```python
from build123d import *

# Parameters (mm, degrees)
SKETCH4_R           = 1.911425658
BOSS_EXTRUDE1_DEPTH = 5.6


with BuildPart() as part:
    # Sketch4 → Boss-Extrude1 (new body)
    with BuildSketch(Plane(origin=(0, 0, 0), x_dir=(1, 0, 0), z_dir=(0, 1, 0))):
        with BuildLine():
            Line((-4, -3.25), (-8.327817762, -2.730391092))
            ThreePointArc((-8.327817762, -2.730391092), (-10.75, 0), (-8.327817762, 2.730391092))
            Line((-8.327817762, 2.730391092), (-4, 3.25))
            Line((-4, 3.25), (4, 3.25))
            Line((4, 3.25), (8.327817762, 2.730391092))
            ThreePointArc((8.327817762, 2.730391092), (10.75, 0), (8.327817762, -2.730391092))
            Line((8.327817762, -2.730391092), (4, -3.25))
            Line((4, -3.25), (-4, -3.25))
        make_face()
        Circle(SKETCH4_R, mode=Mode.SUBTRACT)
    extrude(amount=BOSS_EXTRUDE1_DEPTH)


solid = part.part
```
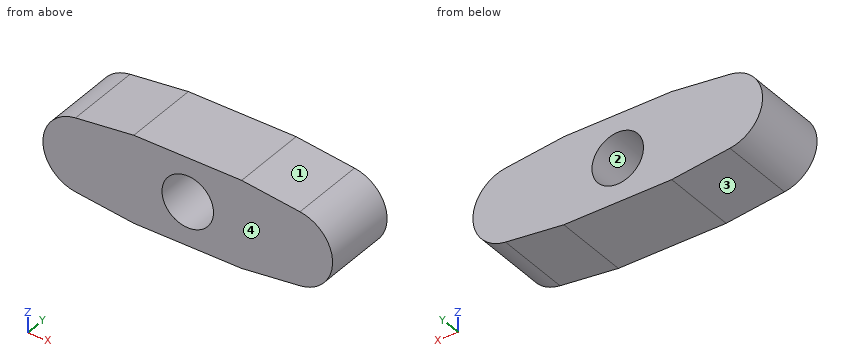
Model file for the job. Use its own axes, mm. Face numbers are marked on the shaded views. Give positions to 0.01 mm unless a question says otherwise; leave off trailing zeros. Loops run counter-clockwise (first coordinate to the right, second up) from the corner with the lowest first, then second, coordinate; pieces in that order, holes last. Notation, with made-up numbers: (32, -0.75) - (86, -0.75) arc R8 cw to (86, 7.25) - close; hole circle Ø4 at (20, -34). An arc over 180 degrees is marked (long way). One line per item, written item: value. Start each with the question number.
1. Probe L1, parallel to Z at x = 0, y = 4.1; L2, parallel to X at y = 1.65, z = 0; L3, parallel to X at y = 3.35, z = -1.25. List the from-to ranges inside material, lowest first. Write a range as from..to.
2. Slice it at A-A (x = 0). List the corners of the cut face in (y, z), plus the area to 3 significant figures.
3. Slice it at C-C (y = 0.6). List the corners of the cut face in (x, z), plus the area to 3 significant figures.
4. Pin check, flat tip, straight feed: pin 1 (2 mm diameter, centred on y = 3, z = 2, fed in from +X). Stop position of the tip, or through.
5. Pull direction X, two halves, no side cores. Call the marked faces 1, 2, 3 and 4: pulls with the +X half, pulls with the -X half, needs draft (parallel to the pull), parting line crosses it, or undercut.
6. Slice it at B-B (z = 0). List the corners of the cut face in (x, y), plus the area to 3 significant figures.
7. Slice it at D-D (z = 2.5). List the corners of the cut face in (x, y).
Solution:
1. L1: z = -3.25..-1.91, 1.91..3.25
1. L2: x = -10.75..-1.91, 1.91..10.75
1. L3: x = -10.45..-1.45, 1.45..10.45
2. outline: (0, -3.25) - (5.6, -3.25) - (5.6, -1.91) - (0, -1.91) - close; (0, 1.91) - (5.6, 1.91) - (5.6, 3.25) - (0, 3.25) - close
2. area: 15.0 mm^2
3. outline: (-8.33, -2.73) - (-4, -3.25) - (4, -3.25) - (8.33, -2.73) arc R2.75 ccw to (8.33, 2.73) - (4, 3.25) - (-4, 3.25) - (-8.33, 2.73) arc R2.75 ccw to start; hole circle Ø3.82 at (0, 0)
3. area: 112 mm^2
4. pin 1: stops at x = 10.56
5. face 1: pulls with the +X half
5. face 2: undercut
5. face 3: pulls with the -X half
5. face 4: needs draft
6. outline: (-10.75, 0) - (-1.91, 0) - (-1.91, 5.6) - (-10.75, 5.6) - close; (1.91, 0) - (10.75, 0) - (10.75, 5.6) - (1.91, 5.6) - close
6. area: 99.0 mm^2
7. outline: (-9.15, 0) - (9.15, 0) - (9.15, 5.6) - (-9.15, 5.6) - close
